For this review, take the finished solid that the model builds, in its own axes (mm). A direction names the side the tool comes from. Round coordinates to 2 decimals unless told otherwise and drop trailing zeros. Write each loop counter-clockwise with the first axis right and the second up, starting at its lowest first coordinate (ties: lowest second). Pieces come first, ordered by that corner, then holes. Notation, with made-up numbers: M 87,-12.75 L 118,-12.75 A14 cw 118,1.25 Z; hole C 21,65.25 d3. An arc over 180 degrees is marked long. Use one line per item in the form item = value. Start each with the question number.
Item 1: For P1, Ø3, axis at x = -6.5, y = -9.5, coming from the -Z side; P2, Ø7, axis at x = 0, y = 0, coming from the -Z side; P3, Ø2, axis at y = 5.5, z = 45.5, coming from the -X side; P4, Ø2.5, axis at x = -1, z = 45.5, coming from the +Y side, all flat-tipped, find the tip position at first contact; note any pin that passes through.
Item 2: Add section A-A (y = 0). State the section outline as (x, z) points.
Item 3: Draft analysis for pull direction X (two halves, no side actions). For faces 4 (the cylindrical face through (-0.1, 5.5, 52.5)), 5 (the cylindrical face through (3.23, -6.21, 42.61)), 6 (the flat face through (2.5, 8, 13)), 7 (the flat face through (2, -7, 33)), state which applies: released by +X, released by -X, zero draft, split by the parting line, or undercut.
Item 4: For line 1 (Y direction, x = 0, z = 12); line 2 (Z direction, x = -3, y = 4.75); line 3 (X direction, y = 6.25, z = 8.5), list the stretches that pass through material, from the lowest coordinate up. Write a range as [from, to].
Item 5: Add section B-B (z = 7). State the section outline as (x, y) points.
Item 6: For faces 1 (the cylindrical face through (-3.23, -6.21, 13.56)), 2 (the flat face through (-2.5, 5, 43)), 3 (the cylindrical face through (11.923, 3.755, 15.79)), list the 3-axis set-ups (+Z, -Z, +X, -X, +Y, -Y) from which the entire face can be reached by the end or side of a thin tool; tool diameter is ignored.
from build123d import *

# Parameters (mm, degrees)
SKETCH_1_R          = 12.5
EXTRUDE_1_DEPTH     = 33
SKETCH_4_R          = 7
EXTRUDE_2_DEPTH     = 3
SKETCH_7_R          = 7
EXTRUDE_3_DEPTH     = 20
CHAMFER_1_SIZE      = 2
CUT_EXTRUDE_4_DEPTH = 3
CHAMFER_2_SIZE      = 0.5
CHAMFER_3_SIZE      = 1
SKETCH_9_R          = 7
CUT_EXTRUDE_5_DEPTH = 28
SKETCH_10_W         = 5
SKETCH_10_H         = 4.667686035
CUT_EXTRUDE_6_DEPTH = 26
CHAMFER_4_SIZE      = 0.5
SKETCH_11_R         = 2.75
CUT_EXTRUDE_7_DEPTH = 50
CHAMFER_5_SIZE      = 0.5
FILLET_1_R          = 1


with BuildPart() as part:
    # 草图1 → 拉伸1 (new body)
    with BuildSketch(Plane.XY):
        Circle(SKETCH_1_R)
    extrude(amount=EXTRUDE_1_DEPTH)

    # 草图4 → 拉伸2 (add)
    with BuildSketch(Plane.XY.offset(33)):
        Circle(SKETCH_4_R)
    extrude(amount=-EXTRUDE_2_DEPTH)

    # 草图7 → 拉伸3 (add)
    with BuildSketch(Plane.XY.offset(33)):
        Circle(SKETCH_7_R)
    extrude(amount=EXTRUDE_3_DEPTH)

    # 倒角1
    chamfer_1_edges = [part.edges().sort_by_distance(p)[0] for p in [
        (-12.5, 0, 33),
    ]]
    chamfer(chamfer_1_edges, length=CHAMFER_1_SIZE)

    # 草图8 → 切除-拉伸4 (cut)
    with BuildSketch(Plane(origin=(0, 7, 0), x_dir=(-1, 0, 0), z_dir=(0, 1, 0))):
        with BuildLine():
            Line((-2.5, 50), (-2.5, 35.5))
            ThreePointArc((-2.5, 35.5), (0, 33), (2.5, 35.5))
            Line((2.5, 35.5), (2.5, 50))
            ThreePointArc((2.5, 50), (0, 52.5), (-2.5, 50))
        make_face()
    extrude(amount=-CUT_EXTRUDE_4_DEPTH, mode=Mode.SUBTRACT)

    # 倒角2
    chamfer_2_edges = [part.edges().sort_by_distance(p)[0] for p in [
        (-7, 0, 53),
    ]]
    chamfer(chamfer_2_edges, length=CHAMFER_2_SIZE - 0.0001)  # a hair under: the kernel refuses the full size

    # 倒角3
    chamfer_3_edges = [part.edges().sort_by_distance(p)[0] for p in [
        (-12.5, 0, 0),
    ]]
    chamfer(chamfer_3_edges, length=CHAMFER_3_SIZE)

    # 草图9 → 切除-拉伸5 (cut)
    with BuildSketch(Plane(origin=(0, 0, 0), x_dir=(-1, 0, 0), z_dir=(0, 0, -1))):
        Circle(SKETCH_9_R)
    extrude(amount=-CUT_EXTRUDE_5_DEPTH, mode=Mode.SUBTRACT)

    # 草图10 → 切除-拉伸6 (cut)
    with BuildSketch(Plane(origin=(0, 0, 0), x_dir=(-1, 0, 0), z_dir=(0, 0, -1))):
        with Locations((0, 6.666156983)):
            Rectangle(SKETCH_10_W, SKETCH_10_H)
    extrude(amount=-CUT_EXTRUDE_6_DEPTH, mode=Mode.SUBTRACT)

    # 倒角4
    chamfer_4_edges = [part.edges().sort_by_distance(p)[0] for p in [
        (3.968626967, -5.766281297, 0),
    ]]
    chamfer(chamfer_4_edges, length=CHAMFER_4_SIZE)

    # 草图11 → 切除-拉伸7 (cut)
    with BuildSketch(Plane.XY.offset(53)):
        Circle(SKETCH_11_R)
    extrude(amount=-CUT_EXTRUDE_7_DEPTH, mode=Mode.SUBTRACT)

    # 倒角5
    chamfer_5_edges = [part.edges().sort_by_distance(p)[0] for p in [
        (-2.75, 0, 53),
    ]]
    chamfer(chamfer_5_edges, length=CHAMFER_5_SIZE)

    # 圆角1
    fillet_1_edges = [part.edges().sort_by_distance(p)[0] for p in [
        (7, 0, 28),
    ]]
    fillet(fillet_1_edges, radius=FILLET_1_R)


solid = part.part
Calculated:
q1.P1 = 0
q1.P2 = 28
q1.P3 = -5.36
q1.P4 = 4
q2.outline = M -12.5,1 L -11.5,0 L -7.5,0 L -7,0.5 L -7,27 A1 cw -6,28 L -2.75,28 L -2.75,52.5 L -3.25,53 L -6.5,53 L -7,52.5 L -7,33 L -10.5,33 L -12.5,31 Z; M 2.75,28 L 6,28 A1 cw 7,27 L 7,0.5 L 7.5,0 L 11.5,0 L 12.5,1 L 12.5,31 L 10.5,33 L 7,33 L 7,52.5 L 6.5,53 L 3.25,53 L 2.75,52.5 Z
q3.face_4 = undercut
q3.face_5 = split by the parting line
q3.face_6 = undercut
q3.face_7 = zero draft
q4.line_1 = [-12.5, -7], [9, 12.5]
q4.line_2 = [28, 53]
q4.line_3 = [-10.83, -3.15], [3.15, 10.83]
q5.outline = C 0,0 d25; hole M -2.5,6.54 A7 ccw long 2.5,6.54 L 2.5,9 L -2.5,9 Z
q6.face_1 = -Z
q6.face_2 = +Y
q6.face_3 = +Z, -Z
